Autodesk Inventor part; units mm, degrees
ref_plane "YZ Plane" through (0, 0, 0) normal (1, 0, 0) x (0, 1, 0)
ref_plane "XZ Plane" through (0, 0, 0) normal (0, 1, 0) x (-1, 0, 0)
ref_plane "XY Plane" through (0, 0, 0) normal (0, 0, 1) x (1, 0, 0)
sketch "Szkic1" plane through (0, 0, 0) normal (0, 0, 1) x (1, 0, 0)
  line L0 (0, -50) -> (2, -50)
  circle A0 centre (-3.1, -7) radius 7
  line L1 (3.9, -50) -> (3.9, 0)
  line L2 (3.9, -50) -> (-19.6026, -42.4936)
  line L3 (2, -14) -> (2, -47.2936)
  line L4 (0, -14) -> (0, -46.6549)
  line L5 (3.9, -47.9005) -> (-27.3591, -37.9167)
  line L6 (-13.8397, -39.3668) -> (-13.1635, -37.9168)
  line L7 (-13.8397, -39.3668) -> (-13.8397, -40.8668)
  line L8 (-13.1635, -37.9168) -> (-16.1635, -37.9168)
  line L9 (-17, -41.2253) -> (-17, 0)
  line L10 (-17, 0) -> (-3.1, 0)
  line L11 (-19, -40.5865) -> (-19, 0.0005)
  line L12 (-19, 0.0005) -> (-3.1, 0.0005)
  line L13 (-3.1, -1.9995) -> (-19, -1.9995)
  line L14 (-19, -1.9995) -> (-19, 0.0005)
  line L15 (-19, -40.5865) -> (-19, -42.6861)
  line L16 (0, -14) -> (0, 0)
  line L17 (2, -14) -> (0, -14)
  line L18 (2, 0) -> (2, -14)
  line L19 (0, 0) -> (2, 0)
  line L20 (-3.1, 0) -> (0, 0)
  line L21 (-3.1, -1.9995) -> (0, -1.9995)
  line L22 (-19, 0.0005) -> (-17, 0.0005)
  line L23 (-17, 0.0005) -> (-17, -1.9995)
  line L24 (-17, -1.9995) -> (-19, -1.9995)
  line L25 (-19, -1.9995) -> (-19, 0.0005)
  dimension "d0" = 2
  dimension "d1" = 1.5
  dimension "d2" = 3
  dimension "d3" = 2
  dimension "d4" = 2
extrude "Wyciągnięcie proste1" add sketch "Szkic1" against normal blind 50 contours L1 L2 L15 L5 | L16 L21 L13 A0 | A0 L20 L16 | A0 L13 L9 L10 | L9 L13 L11 L12 | L9 L5 L11 L13 picked at (-1.3641, -1.4413)
sketch "Szkic3" plane through (0, 0, -50) normal (0, 0, -1) x (-1, 0, 0)
  line L0 (17, -1.9995) -> (17, -41.2253)
  line L1 (17, -41.2253) -> (-3.9, -47.9005)
  line L2 (-3.9, -47.9005) -> (-3.9, -50)
  line L3 (-3.9, -50) -> (19, -42.6861)
  line L4 (19, -42.6861) -> (19, 0.0005)
  line L5 (19, 0.0005) -> (17, 0.0005)
  line L6 (17, 0.0005) -> (17, 0)
  line L7 (17, 0) -> (0, 0)
  line L8 (0, 0) -> (0, -1.9995)
  line L9 (0, -1.9995) -> (17, -1.9995)
  line L10 (12.25, 0) -> (12.25, -47.2936)
  line L11 (12.25, -47.2936) -> (13.85, -47.2936)
  line L12 (13.85, 0) -> (13.85, -47.2936)
  line L13 (12.25, 0) -> (13.85, 0)
  point P0 (13.85, -42.2314)
  point P1 (13.85, -44.3309)
extrude "Wyciągnięcie proste3" cut sketch "Szkic3" against normal through all contours L9 L12 L7 L5 L4 L3 L1 L0 | L9 L10 L7 L12 | L9 L8 L7 L10
sketch "Szkic4" plane through (0, 0, -50) normal (0, 0, -1) x (-1, 0, 0)
  line L0 (13.85, -44.3309) -> (13.85, -42.2314)
  line L1 (13.85, -42.2314) -> (-3.9, -47.9005)
  line L2 (-3.9, -47.9005) -> (-3.9, -50)
  line L3 (-3.9, -50) -> (13.85, -44.3309)
  line L4 (13.85, -42.2314) -> (16.85, -41.2732)
  line L5 (16.85, -41.2732) -> (16.85, -43.3727)
  line L6 (16.85, -43.3727) -> (13.85, -44.3309)
  point P0 (0, 0)
  dimension "d12" = 3
extrude "Wyciągnięcie proste4" add sketch "Szkic4" against normal blind 50 contours L0 L4 L5 L6
properties part number "nozzz" material "Stal, węglowa"
Work out the finished part from the listing and answer in its coordinate system (mm). Coordinates: 2 decimals unless noted, no trailing zeros. Loops run counter-clockwise (first coordinate to the right, second up) from the corner with the lowest first, then second, coordinate; pieces in that order, holes last. Notation, with made-up numbers: (80, -25.75) -> (130, -25.75) arc R22 cw to (130, -6.75) -> close; hole circle Ø3 at (-20, -4). An arc over 180 degrees is marked (long way). Write each question's results on one line, items separated by ' | '. Start each with the question number.
1) Find section B-B on x = -1.25. Determine the outline of the cut face in (y, z), then the cut area to 3 significant figures.
2) Consider line 1 along Y through (x, z) = (-13.75, -23); line 2 along Y through (x, z) = (-0.25, -39.5). Determine where each line is inside the solid, lowest interval first.
3) Find section A-A on z = -9. Determine the outline of the cut face in (x, y).
4) Flat-ended cylindrical pins translate along their axes: P1, Ø2, axis at y = -47, z = -6, coming from the +X side; P2, Ø3, axis at x = -0.5, z = -34, coming from the +Y side; P3, Ø1.5, axis at x = -3.5, z = -25, coming from the -Y side; P4, Ø2, axis at x = -13, z = -37.5, coming from the -Y side. Find the tip coordinate at first contact, or state that the pin passes through.
5) Find section C-C on y = -45. Determine the outline of the cut face in (x, z), then the cut area to 3 significant figures.
Response values:
1) outline: (-48.36, -50) -> (-46.26, -50) -> (-46.26, 0) -> (-48.36, 0) -> close | area: 105 mm^2
2) line 1: y = -44.36 to -42.26 | line 2: y = -48.67 to -46.58
3) outline: (-16.85, -43.37) -> (-13.85, -44.33) -> (3.9, -50) -> (3.9, -47.9) -> (-13.85, -42.23) -> (-16.85, -41.27) -> close
4) P1: stops at x = 3.9 | P2: stops at y = -46.02 | P3: stops at y = -47.88 | P4: stops at y = -44.92
5) outline: (-11.76, -50) -> (-5.18, -50) -> (-5.18, 0) -> (-11.76, 0) -> close | area: 329 mm^2
